The model under review builds one solid part; all positions refer to its coordinate system, in mm. Coordinates: 2 decimals unless noted, no trailing zeros. Order: outer loops, then holes, each group sorted by start corner. A loop starts at its lowest first (then second) coordinate and runs counter-clockwise, first axis right, second up. Notation, with made-up numbers: (-20.75, 80) -> (0.25, 80) arc R34 ccw to (0.25, 113) -> close; hole circle Ø5 at (-12, 18). An arc over 180 degrees is marked (long way). Put each result on its own line as item: value.
from build123d import *

# Parameters (mm, degrees)
BOSS_EXTRUDE1_DEPTH      = 2.3876
BOSS_EXTRUDE1_DEPTH_BACK = 2.3876
SKETCH4_R                = 3.2639
CUT_EXTRUDE1_DEPTH       = 5.7752


with BuildPart() as part:
    # Sketch3 → Boss-Extrude1 (new body, two sides)
    with BuildSketch(Plane.XY) as boss_extrude1_sk:
        Polygon((50.8, -50.8), (-50.8, -50.8), (-50.8, -25.4), (-12.7, 50.8), (12.7, 50.8), (50.8, -25.4), align=None)
    extrude(amount=BOSS_EXTRUDE1_DEPTH)
    extrude(boss_extrude1_sk.sketch, amount=-BOSS_EXTRUDE1_DEPTH_BACK)

    # Sketch4 → Cut-Extrude1 (cut, through all)
    with BuildSketch(Plane.XY.offset(2.3876)):
        with Locations((-38.1, -38.1)):
            Circle(SKETCH4_R)
        with Locations((-12.7, -38.1)):
            Circle(SKETCH4_R)
        with Locations((12.7, -38.1)):
            Circle(SKETCH4_R)
        with Locations((0, 38.1)):
            Circle(SKETCH4_R)
        with Locations((0, 12.7)):
            Circle(SKETCH4_R)
        with Locations((38.1, -38.1)):
            Circle(SKETCH4_R)
        with Locations((0, -12.7)):
            Circle(SKETCH4_R)
    extrude(amount=-CUT_EXTRUDE1_DEPTH, mode=Mode.SUBTRACT)


solid = part.part
Item 1: For pin 1 Ø6 at (x, y) = (0, -12.7) entering from +Z; pin 2 Ø1.5 at (y, z) = (21.5, 2) entering from -X (3 decimals), all flat-tipped, find the tip position at first contact; note any pin that passes through.
Answers below:
pin 1: through
pin 2: x = -27.725
Item 2: Consider section B-B on y = -12.7. Write out the cut boundary in (x, z).
Answers below:
outline: (-44.45, -2.39) -> (-3.26, -2.39) -> (-3.26, 2.39) -> (-44.45, 2.39) -> close; (3.26, -2.39) -> (44.45, -2.39) -> (44.45, 2.39) -> (3.26, 2.39) -> close
Item 3: Mouldability with a two-part tool opening along X and no side actions: class faces 1 (the flat face through (-50.8, -38, 0)), 2 (the cylindrical face through (-0.425, -9.464, 0.033)), 3 (the flat face through (1, -50.8, 0)) as +X half, -X half, draft (parallel to the pull), parting line (faces both ways), or undercut.
Answers below:
face 1: -X half
face 2: undercut
face 3: draft
Item 4: For line 1 (Y direction, x = -12.7, z = 0.3); line 2 (Y direction, x = 0, z = 0.8); line 3 (Y direction, x = 0.5, z = -0.25), list the stretches that pass through material, from the lowest coordinate up. Write a range as from..to.
Answers below:
line 1: -50.8..-41.36, -34.84..50.8
line 2: -50.8..-15.96, -9.44..9.44, 15.96..34.84, 41.36..50.8
line 3: -50.8..-15.93, -9.47..9.47, 15.93..34.87, 41.33..50.8
Item 5: Consider section A-A on x = -38.1. Write out the cut boundary in (y, z).
Answers below:
outline: (-50.8, -2.39) -> (-41.36, -2.39) -> (-41.36, 2.39) -> (-50.8, 2.39) -> close; (-34.84, -2.39) -> (0, -2.39) -> (0, 2.39) -> (-34.84, 2.39) -> close
Item 6: Consider section D-D on y = -38.1. Write out the cut boundary in (x, z), and give its area (3 significant figures).
Answers below:
outline: (-50.8, -2.39) -> (-41.36, -2.39) -> (-41.36, 2.39) -> (-50.8, 2.39) -> close; (-34.84, -2.39) -> (-15.96, -2.39) -> (-15.96, 2.39) -> (-34.84, 2.39) -> close; (-9.44, -2.39) -> (9.44, -2.39) -> (9.44, 2.39) -> (-9.44, 2.39) -> close; (15.96, -2.39) -> (34.84, -2.39) -> (34.84, 2.39) -> (15.96, 2.39) -> close; (41.36, -2.39) -> (50.8, -2.39) -> (50.8, 2.39) -> (41.36, 2.39) -> close
area: 360 mm^2
Item 7: Consider section C-C on x = 0. Write out the cut boundary in (y, z).
Answers below:
outline: (-50.8, -2.39) -> (-15.96, -2.39) -> (-15.96, 2.39) -> (-50.8, 2.39) -> close; (-9.44, -2.39) -> (9.44, -2.39) -> (9.44, 2.39) -> (-9.44, 2.39) -> close; (15.96, -2.39) -> (34.84, -2.39) -> (34.84, 2.39) -> (15.96, 2.39) -> close; (41.36, -2.39) -> (50.8, -2.39) -> (50.8, 2.39) -> (41.36, 2.39) -> close
